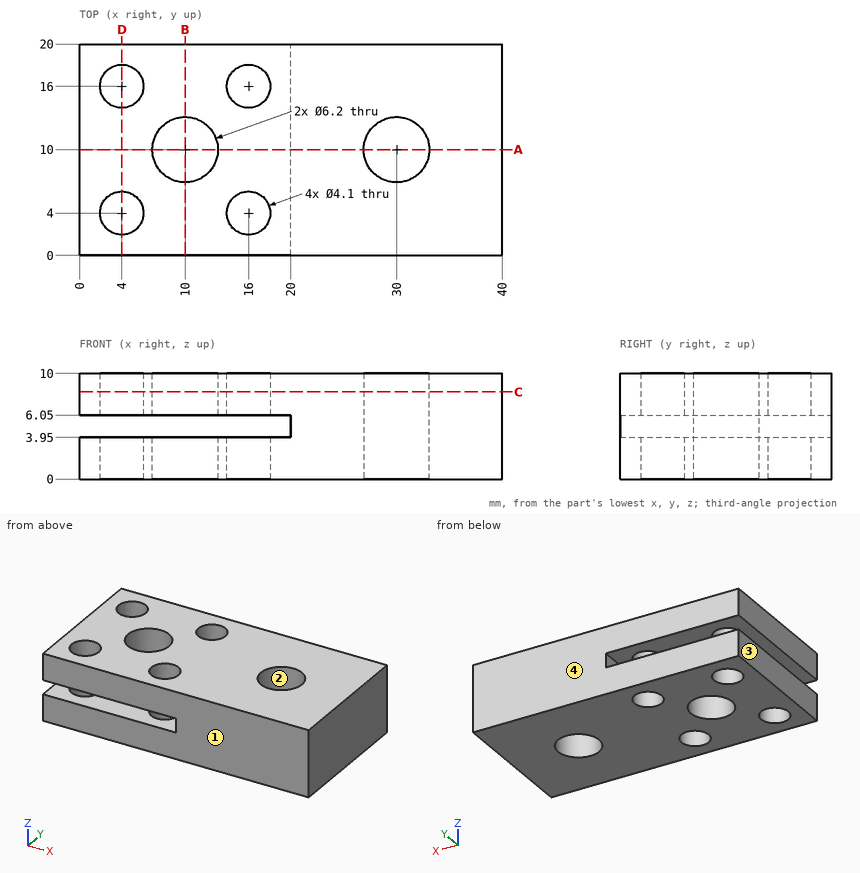
Input: dimensioned drawing with shaded views. Units: mm. Origin: part minimum x, y, z. Give positions to 0.01 mm unless a question says otherwise; leave off trailing zeros. Write each loop counter-clockwise with the first axis right and the second up, starting at its lowest first coordinate (ties: lowest second). Pieces come first, ordered by that corner, then holes.
1. Line query: probe 1 along Z at (x, y) = (18.5, 15); probe 2 along Y at (x, z) = (5, 1); probe 3 along X at (y, z) = (17.75, 2.75). Output: solid intervals per line, ascending.
2. Section query D-D, the plane x = 4. Return loops of the section in (y, z).
3. Draft query along Y for the marked faces 1, 2, 3 and 4. Return one class per face: released by +Y, released by -Y, zero draft, split by the parting line, or undercut.
4. Section query B-B, the plane x = 10. Return loops of the section in (y, z), then the cut area to 3 significant figures.
5. Section query A-A, the plane y = 10. Return loops of the section in (x, z).
6. Section query C-C, the plane z = 8.25. Return loops of the section in (x, y).
Computed:
1. probe 1: z = 0 to 3.95, 6.05 to 10
1. probe 2: y = 0 to 2.21, 5.79 to 14.21, 17.79 to 20
1. probe 3: x = 0 to 2.93, 5.07 to 14.93, 17.07 to 40
2. outline: (0, 0) - (1.95, 0) - (1.95, 3.95) - (0, 3.95) - close; (0, 6.05) - (1.95, 6.05) - (1.95, 10) - (0, 10) - close; (6.05, 0) - (13.95, 0) - (13.95, 3.95) - (6.05, 3.95) - close; (6.05, 6.05) - (13.95, 6.05) - (13.95, 10) - (6.05, 10) - close; (18.05, 0) - (20, 0) - (20, 3.95) - (18.05, 3.95) - close; (18.05, 6.05) - (20, 6.05) - (20, 10) - (18.05, 10) - close
3. face 1: released by -Y
3. face 2: undercut
3. face 3: zero draft
3. face 4: released by +Y
4. outline: (0, 0) - (6.9, 0) - (6.9, 3.95) - (0, 3.95) - close; (0, 6.05) - (6.9, 6.05) - (6.9, 10) - (0, 10) - close; (13.1, 0) - (20, 0) - (20, 3.95) - (13.1, 3.95) - close; (13.1, 6.05) - (20, 6.05) - (20, 10) - (13.1, 10) - close
4. area: 109 mm2
5. outline: (0, 0) - (6.9, 0) - (6.9, 3.95) - (0, 3.95) - close; (0, 6.05) - (6.9, 6.05) - (6.9, 10) - (0, 10) - close; (13.1, 0) - (26.9, 0) - (26.9, 10) - (13.1, 10) - (13.1, 6.05) - (20, 6.05) - (20, 3.95) - (13.1, 3.95) - close; (33.1, 0) - (40, 0) - (40, 10) - (33.1, 10) - close
6. outline: (0, 0) - (40, 0) - (40, 20) - (0, 20) - close; hole circle Ø4.1 at (4, 4); hole circle Ø4.1 at (4, 16); hole circle Ø6.2 at (10, 10); hole circle Ø4.1 at (16, 4); hole circle Ø4.1 at (16, 16); hole circle Ø6.2 at (30, 10)
